The model under review builds one solid part; all positions refer to its coordinate system, in mm. Coordinates: 2 decimals unless noted, no trailing zeros. Order: outer loops, then holes, each group sorted by start corner. A loop starts at its lowest first (then second) coordinate and runs counter-clockwise, first axis right, second up. Notation, with made-up numbers: M -16.5,27.25 L 25.5,27.25 A24 cw 25.5,59.25 Z; hole C -14,14 d11. An arc over 180 degrees is marked long. Write each question's results on one line, items separated by ' | '.
from build123d import *

# Parameters (mm, degrees)
SKETCH1_W           = 200
SKETCH1_H           = 40
BOSS_EXTRUDE1_DEPTH = 2
SKETCH2_W           = 6.740804159
SKETCH2_H           = 2
SKETCH2_R           = 0.5
BOSS_EXTRUDE2_DEPTH = 2
BOSS_EXTRUDE3_START = 2
SKETCH3_W           = 6
SKETCH3_H           = 2
SKETCH3_R           = 0.5
BOSS_EXTRUDE3_DEPTH = 2
SKETCH4_R           = 0.5
CUT_EXTRUDE1_DEPTH  = 204.204330663
FILLET2_R           = 1


with BuildPart() as part:
    # Sketch1 → Boss-Extrude1 (new body)
    with BuildSketch(Plane(origin=(0, 0, 0), x_dir=(1, 0, 0), z_dir=(0, 1, 0))):
        Rectangle(SKETCH1_W, SKETCH1_H)
    extrude(amount=BOSS_EXTRUDE1_DEPTH)

    # Sketch2 → Boss-Extrude2 (add)
    with BuildSketch(Plane(origin=(100, 0, 0), x_dir=(0, 0, -1), z_dir=(1, 0, 0))):
        with Locations((-18.629597921, 1)):
            Rectangle(SKETCH2_W, SKETCH2_H)
        with Locations((-21, 1)):
            Circle(SKETCH2_R, mode=Mode.SUBTRACT)
    extrude(amount=BOSS_EXTRUDE2_DEPTH)

    # Sketch3 → Boss-Extrude3 (add)
    with BuildSketch(Plane.ZY.offset(100).offset(BOSS_EXTRUDE3_START)):
        with Locations((19, 1)):
            Rectangle(SKETCH3_W, SKETCH3_H)
        with Locations(Location((21, 1, 0), (0, 0, 180))):
            Circle(SKETCH3_R, mode=Mode.SUBTRACT)
    extrude(amount=-BOSS_EXTRUDE3_DEPTH)

    # Sketch4 → Cut-Extrude1 (cut, through all)
    with BuildSketch(Plane.ZY.offset(100)):
        with Locations((-19, 1)):
            Circle(SKETCH4_R)
    extrude(amount=-CUT_EXTRUDE1_DEPTH, mode=Mode.SUBTRACT)

    # Fillet2
    fillet2_edges = [part.edges().sort_by_distance(p)[0] for p in [
        (0, 0, -20),
        (0, 2, -20),
    ]]
    fillet(fillet2_edges, radius=FILLET2_R - 0.0001)  # a hair under: the kernel refuses the full size


solid = part.part
1) Take a section at B-B on z = -15. State the section outline as (x, y) points, plus the area to 3 significant figures.
Solutions:
outline: M -100,0 L 100,0 L 100,2 L -100,2 Z | area: 400 mm2
2) For pin 1 (0.6 mm diameter, centred on y = 1, z = -3, fed in from +X); pin 2 (1 mm diameter, centred on y = 1.5, z = -11.5, fed in from -X), all flat-tipped, find the tip position at first contact; note any pin that passes through.
Solutions:
pin 1: x = 100 | pin 2: x = -100
3) To check wall thickness, follow line 1 along Z through (x, y) = (-100.6, 1); line 2 along Y through (x, z) = (101.65, 21); line 3 along Z through (x, y) = (-30.5, 1.05). State the ranges of each line that lie inside material, in increasing order.
Solutions:
line 1: 16 to 20.5, 21.5 to 22 | line 2: 0 to 0.5, 1.5 to 2 | line 3: -20 to -19.5, -18.5 to 20
